```python
from build123d import *

# Parameters (mm, degrees)
CROQUIS1_R              = 1.5
CROQUIS1_R_2            = 4
CROQUIS1_R_3            = 4.5
SALIENTE_EXTRUIR1_DEPTH = 6


with BuildPart() as part:
    # Croquis1 → Saliente-Extruir1 (new body)
    with BuildSketch(Plane.XY):
        with BuildLine():
            ThreePointArc((-153.452479084, 65.245629882), (-149.916945178, 66.710095976), (-148.452479084, 70.245629882))
            Line((-148.452479084, 70.245629882), (-148.452479084, 77.241660705))
            ThreePointArc((-148.452479084, 77.241660705), (-149.261781775, 79.96894068), (-151.427701509, 81.813342646))
            Line((-151.427701509, 81.813342646), (-176.86343393, 93.078715272))
            ThreePointArc((-176.86343393, 93.078715272), (-177.372149016, 93.339780675), (-177.847731471, 93.657219664))
            Line((-177.847731471, 93.657219663), (-243.282498112, 142.965853083))
            ThreePointArc((-243.282498112, 142.965853083), (-245.323514753, 145.031918552), (-246.684791002, 147.597323475))
            ThreePointArc((-246.684791002, 147.597323475), (-249.33333249, 155.226277836), (-253.46024382, 162.167770437))
            ThreePointArc((-253.46024382, 162.167770437), (-255.706791789, 164.36963499), (-258.526200935, 165.764668091))
            ThreePointArc((-258.526200935, 165.764668091), (-267.807267276, 167.484933762), (-277.233031605, 166.98246665))
            ThreePointArc((-277.233031605, 166.98246665), (-280.839635864, 165.006508056), (-281.744934312, 160.994969527))
            ThreePointArc((-281.744934312, 160.994969527), (-279.629843944, 151.795844616), (-275.418009863, 143.348480526))
            ThreePointArc((-275.418009863, 143.348480526), (-273.299883496, 141.022813744), (-270.564082899, 139.470209357))
            ThreePointArc((-270.564082899, 139.470209357), (-262.753961023, 137.416502238), (-254.690502443, 136.973385563))
            ThreePointArc((-254.690502443, 136.973385563), (-251.84925837, 136.371964278), (-249.300648344, 134.979497983))
            Line((-249.300648344, 134.979497983), (-183.81253652, 85.630666085))
            ThreePointArc((-183.81253652, 85.630666085), (-183.561856018, 85.428793496), (-183.324683063, 85.211210762))
            Line((-183.324683063, 85.211210762), (-164.378251009, 66.671907655))
            ThreePointArc((-164.378251009, 66.671907655), (-162.769627082, 65.615910067), (-160.881322437, 65.245629882))
            Line((-160.881322437, 65.245629882), (-153.452479084, 65.245629882))
        make_face()
        with Locations((-156.438834184, 71.263780114)):
            Circle(CROQUIS1_R, mode=Mode.SUBTRACT)
        with Locations((-174.012762489, 84.506684964)):
            Circle(CROQUIS1_R, mode=Mode.SUBTRACT)
        with Locations((-163.702479084, 80.495629882)):
            Circle(CROQUIS1_R_2, mode=Mode.SUBTRACT)
        with Locations((-192.377432136, 98.345456156)):
            Circle(CROQUIS1_R, mode=Mode.SUBTRACT)
        with BuildLine():
            Line((-271.680758131, 150.180525793), (-274.453508724, 149.79084111))
            ThreePointArc((-274.453508724, 149.79084111), (-276.147670478, 151.067483562), (-274.871028026, 152.761645316))
            Line((-274.871028026, 152.761645316), (-272.098277434, 153.151329999))
            ThreePointArc((-272.098277434, 153.151329999), (-270.404115679, 151.874687547), (-271.680758131, 150.180525793))
        make_face(mode=Mode.SUBTRACT)
        with BuildLine():
            Line((-261.989778965, 145.534030037), (-261.600094282, 142.761279445))
            ThreePointArc((-261.600094282, 142.761279445), (-262.876736734, 141.06711769), (-264.570898489, 142.343760142))
            Line((-264.570898489, 142.343760142), (-264.960583171, 145.116510734))
            ThreePointArc((-264.960583171, 145.116510734), (-263.68394072, 146.810672489), (-261.989778965, 145.534030037))
        make_face(mode=Mode.SUBTRACT)
        with Locations((-264.51202067, 152.702767498)):
            Circle(CROQUIS1_R_3, mode=Mode.SUBTRACT)
        with BuildLine():
            Line((-257.34328321, 155.225009203), (-254.570532617, 155.614693886))
            ThreePointArc((-254.570532617, 155.614693886), (-252.876370863, 154.338051434), (-254.153013314, 152.64388968))
            Line((-254.153013314, 152.64388968), (-256.925763907, 152.254204997))
            ThreePointArc((-256.925763907, 152.254204997), (-258.619925661, 153.530847449), (-257.34328321, 155.225009203))
        make_face(mode=Mode.SUBTRACT)
        with Locations((-274.894282301, 160.526362799)):
            Circle(CROQUIS1_R_2, mode=Mode.SUBTRACT)
        with BuildLine():
            Line((-267.034262376, 159.871504959), (-267.423947058, 162.644255551))
            ThreePointArc((-267.423947058, 162.644255551), (-266.147304607, 164.338417306), (-264.453142852, 163.061774854))
            Line((-264.453142852, 163.061774854), (-264.063458169, 160.289024262))
            ThreePointArc((-264.063458169, 160.289024262), (-265.340100621, 158.594862507), (-267.034262376, 159.871504959))
        make_face(mode=Mode.SUBTRACT)
    extrude(amount=SALIENTE_EXTRUIR1_DEPTH)


solid = part.part
```
Could you check a few things on this model? Use its own coordinates, in mm. A direction names the side the tool comes from. Round coordinates to 2 decimals unless told otherwise and drop trailing zeros. Loops run counter-clockwise (first coordinate to the right, second up) from the corner with the lowest first, then second, coordinate; pieces in that order, holes last.
Q1. Please list where these lines run through material, in increasing order: L1, parallel to Y at x = -264, z = 1.4; L2, parallel to Y at x = -164.5, z = 3.35; L3, parallel to X at y = 82, z = 5.65.
Q2. I want a section at C-C (y = 128.5). Write out the boundary of the cut face in (x, z), and give its area (3 significant figures).
Q3. I want a section at B-B (z = 1.8). Give the number of separate pieces and of enclosed holes in the cut face, and give its area (3 significant figures).
Q4. For P1, Ø3, axis at x = -171.5, z = 0.5, coming from the +Y side; P2, Ø10, axis at x = -231, y = 114, coming from the -Z side; P3, Ø4, axis at x = -156.44, y = 71.26, coming from the -Z side; P4, Ø1, axis at y = 94, z = 4, coming from the -X side, each with a flat end and sliding along its axis, tell me the tip position at first contact or that it passes through.
Q5. On a 3-axis mill with a long thin cutter (end or side, diameter ignored), from which of +Z, -Z, +X, -X, +Y, -Y can I reach the whole of each face in a straight line? I mean faces 4 (the flat face through (-255.976, 155.417, 2.958)), 5 (the cylindrical face through (-149.96, 66.67, 2.96)). Say none if no direction works.
Q6. I want a section at A-A (x = -227). Write out the boundary of the cut face in (y, z).
Q7. Thinking about a two-plate mould opening in X: for faces 1 (the flat face through (-267.226, 161.238, 2.958)), 2 (the cylindrical face through (-245.3, 145, 3)), 3 (the cylindrical face through (-162.795, 65.626, 2.958)), which applies, pulls with the +X half, pulls with the -X half, needs draft (parallel to the pull), parting line crosses it, or undercut?
Answer below:
1. L1: y = 137.63 to 141.36, 146.73 to 148.23, 157.17 to 167.05
1. L2: y = 66.79 to 76.58, 84.42 to 87.6
1. L3: x = -180.04 to -167.41, -160 to -151.85
2. outline: (-240.7, 0) - (-224.09, 0) - (-224.09, 6) - (-240.7, 6) - close
2. area: 99.7 mm2
3. separate pieces: 1
3. enclosed holes: 10
3. area: 2,010 mm2
4. P1: stops at y = 91.37
4. P2: passes through
4. P3: stops at z = 0
4. P4: stops at x = -195.58
5. face 4: +Z, -Z
5. face 5: +Z, -Z, +X, -Y
6. outline: (118.17, 0) - (130.7, 0) - (130.7, 6) - (118.17, 6) - close
7. face 1: undercut
7. face 2: pulls with the +X half
7. face 3: pulls with the -X half
